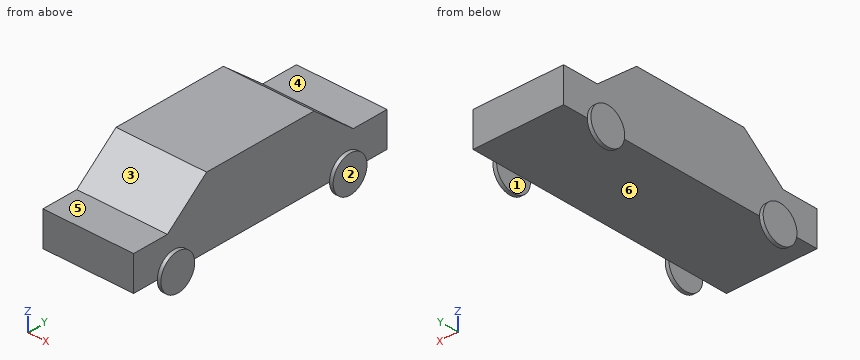
from build123d import *

# Parameters (mm, degrees)
F0_W     = 25
F0_H     = 37.5
F1_DEPTH = 19
F2_R     = 5
F3_DEPTH = 1
F5_DEPTH = 25.001


with BuildPart() as f1:
    # F0 (on Top) → F1 (new body)
    with BuildSketch(Plane.XY):
        with Locations((0, 18.75)):
            Rectangle(F0_W, F0_H)
    extrude(amount=F1_DEPTH)

    # F4 (on face) → F5 (cut, through all)
    with BuildSketch(Plane.YZ.offset(12.5)):
        Polygon((27.5, 9.5), (37.5, 9.5), (37.5, 19), (15.8918132338, 19), align=None)
    extrude(amount=-F5_DEPTH, mode=Mode.SUBTRACT)



with BuildPart() as f3:
    # F2 (on face) → F3 (new body)
    with BuildSketch(Plane.YZ.offset(12.5)):
        with Locations((25.5, 0)):
            Circle(F2_R)
    extrude(amount=F3_DEPTH)


with BuildPart() as f1_1:
    add(f1.part)

    add(f3.part)  # F6 merges F3
    # F6: F1, F3 across plane
    add(f1.part.mirror(Plane.YZ))
    add(f3.part.mirror(Plane.YZ))

    # F7: F1 across plane


with BuildPart() as f1_2:
    add(f1_1.part)
    add(f1_1.part.mirror(Plane.XZ))


solid = f1_2.part
Source: CAD feature listing. Evaluate the final solid. Frame: model axes, mm. Face numbers are marked on the shaded views. A direction names the side the tool comes from. Coordinates: 2 decimals unless noted, no trailing zeros. Loops run counter-clockwise (first coordinate to the right, second up) from the corner with the lowest first, then second, coordinate; pieces in that order, holes last. Notation, with made-up numbers: M 28,46 L 45,46 A33 ccw 45,76 Z; hole C 43.25,0 d10. An arc over 180 degrees is marked long. Answer in a Markdown table with one row per item.
Q1. Section A-A on x = -9.75. Return the cut outline in (y, z), plus the area to 3 significant figures.
Answers below:
| item | result |
|---|---|
| outline | M -37.5,0 L 37.5,0 L 37.5,9.5 L 27.5,9.5 L 15.89,19 L -15.89,19 L -27.5,9.5 L -37.5,9.5 Z |
| area | 1,120 mm^2 |
Q2. First-contact query: pin 1 (1 mm diameter, centred on y = 1, z = 0, fed in from +X); pin 2 (1 mm diameter, centred on y = 4.5, z = 5, fed in from -X); pin 3 (7.5 mm diameter, centred on x = 3, y = -13, fed in from -Z); pin 4 (5 mm diameter, centred on x = -8.5, z = -0.5, fed in from +Y). Flat tips, straight axial feed; report the tip coordinate or a pass-through.
Answers below:
| item | result |
|---|---|
| pin 1 | stops at x = 12.5 |
| pin 2 | stops at x = -12.5 |
| pin 3 | stops at z = 0 |
| pin 4 | stops at y = 37.5 |
Q3. Section B-B on y = -25.5. Return the cut outline in (x, z).
Answers below:
| item | result |
|---|---|
| outline | M -13.5,-5 L -12.5,-5 L -12.5,0 L 12.5,0 L 12.5,-5 L 13.5,-5 L 13.5,5 L 12.5,5 L 12.5,11.14 L -12.5,11.14 L -12.5,5 L -13.5,5 Z |
Q4. Section D-D on z = 13.5. Return the cut outline in (x, y), plus the area to 3 significant figures.
Answers below:
| item | result |
|---|---|
| outline | M -12.5,-22.61 L 12.5,-22.61 L 12.5,22.61 L -12.5,22.61 Z |
| area | 1,130 mm^2 |
Q5. Draft query along X for the marked faces 1, 2 and 3. Return one class per face: pulls with the +X half, pulls with the -X half, needs draft (parallel to the pull), parting line crosses it, or undercut.
Answers below:
| item | result |
|---|---|
| face 1 | undercut |
| face 2 | pulls with the +X half |
| face 3 | needs draft |
Q6. Ray query, probe 1 along X at (y, z) = (27, -0.25); probe 2 along X at (y, z) = (-3, 8); probe 3 along Z at (x, y) = (9.5, -13.5). Return the intervals inside material, ascending. Write a range as from..to.
Answers below:
| item | result |
|---|---|
| probe 1 | x = -13.5..-12.5, 12.5..13.5 |
| probe 2 | x = -12.5..12.5 |
| probe 3 | z = 0..19 |
Q7. Set-up query: the marked faces 4, 5 and 6. Return all of +Z, -Z, +X, -X, +Y, -Y with unobstructed straight access to the full face (end or side cutting, diameter ignored); none if empty.
Answers below:
| item | result |
|---|---|
| face 4 | +Z, +X, -X, +Y |
| face 5 | +Z, +X, -X, -Y |
| face 6 | -Z, +Y, -Y |
Q8. Section C-C on z = -3.5. Return the cut outline in (x, y).
Answers below:
| item | result |
|---|---|
| outline | M -13.5,-29.07 L -12.5,-29.07 L -12.5,-21.93 L -13.5,-21.93 Z; M -13.5,21.93 L -12.5,21.93 L -12.5,29.07 L -13.5,29.07 Z; M 12.5,-29.07 L 13.5,-29.07 L 13.5,-21.93 L 12.5,-21.93 Z; M 12.5,21.93 L 13.5,21.93 L 13.5,29.07 L 12.5,29.07 Z |
